Job drawing, mm, ordinate dimensions from the low corner. One solid piece. A direction names the side the tool comes from. Coordinates: 2 decimals unless noted, no trailing zeros. Write each loop counter-clockwise with the first axis right and the second up, starting at its lowest first coordinate (ties: lowest second). Pieces come first, ordered by that corner, then holes. Notation, with made-up numbers: (34.25, 49) -> (87.25, 49) arc R9 ccw to (87.25, 58) -> close; hole circle Ø7 at (-3.75, -38.5). An arc over 180 degrees is marked (long way). One line per question, with ' | ' between items. Start each with the question number.
Item 1: Saw through at B-B (z = 20). List the corners of the cut face in (x, y), and give its area (3 significant figures).
Item 2: Saw through at D-D (y = 4.5). List the corners of the cut face in (x, z), and give its area (3 significant figures).
Item 3: Two-plate mould, pull along Z, no slides. Class the marked faces 3, 4 and 5: pulls with the +Z half, pulls with the -Z half, needs draft (parallel to the pull), parting line crosses it, or undercut.
Item 4: Pin check, flat tips, straight feed: pin 1 (7 mm diameter, centred on x = 15, z = 20, fed in from +Y); pin 2 (2.5 mm diameter, centred on x = 89.5, y = 13.5, fed in from -Z); pin 3 (3.5 mm diameter, centred on x = 15, z = 20, fed in from -Y); pin 4 (4 mm diameter, centred on x = 129.5, z = 18, fed in from +Y). Stop position of each tip, or through.
Item 5: Probe probe 1 along Z at (x, y) = (74.5, 19); probe 2 along X at (y, z) = (9.25, 9); probe 3 along X at (y, z) = (17.5, 17.5). List the from-to ranges inside material, lowest first. Write a range as [from, to].
Item 6: Saw through at C-C (x = 135). List the corners of the cut face in (y, z), and give its area (3 significant figures).
Item 7: 3-axis set-ups, long thin cutter, end or side, ignore diameter. For the marked faces 1 and 2: which of +Z, -Z, +X, -X, +Y, -Y reach the whole face in a straight line?
Item 8: Saw through at A-A (y = 13.5). List the corners of the cut face in (x, z), and give its area (3 significant figures).
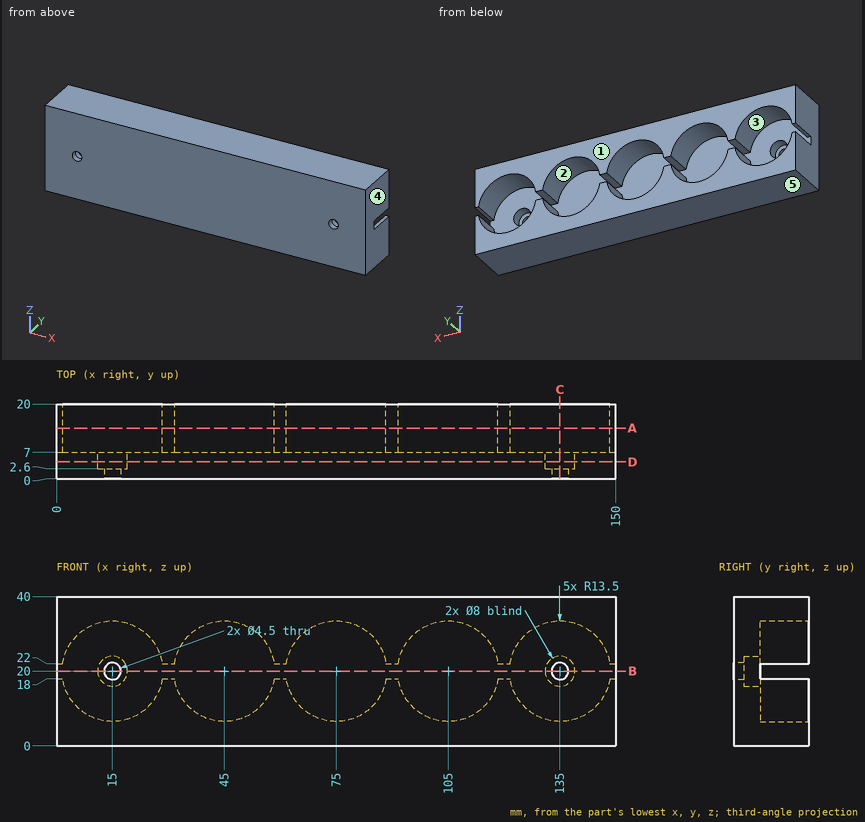
From the geometry:
1) outline: (0, 0) -> (12.75, 0) -> (12.75, 2.6) -> (11, 2.6) -> (11, 7) -> (0, 7) -> close; (17.25, 0) -> (132.75, 0) -> (132.75, 2.6) -> (131, 2.6) -> (131, 7) -> (19, 7) -> (19, 2.6) -> (17.25, 2.6) -> close; (137.25, 0) -> (150, 0) -> (150, 7) -> (139, 7) -> (139, 2.6) -> (137.25, 2.6) -> close | area: 956 mm2
2) outline: (0, 0) -> (150, 0) -> (150, 40) -> (0, 40) -> close; hole circle Ø8 at (15, 20); hole circle Ø8 at (135, 20) | area: 5,900 mm2
3) face 3: undercut | face 4: needs draft | face 5: pulls with the -Z half
4) pin 1: y = 2.6 | pin 2: z = 0 | pin 3: through | pin 4: y = 7
5) probe 1: [0, 6.51], [33.49, 40] | probe 2: [0, 7.17], [22.83, 37.17], [52.83, 67.17], [82.83, 97.17], [112.83, 127.17], [142.83, 150] | probe 3: [0, 1.73], [28.27, 31.73], [58.27, 61.73], [88.27, 91.73], [118.27, 121.73], [148.27, 150]
6) outline: (0, 0) -> (20, 0) -> (20, 6.5) -> (7, 6.5) -> (7, 16) -> (2.6, 16) -> (2.6, 17.75) -> (0, 17.75) -> close; (0, 22.25) -> (2.6, 22.25) -> (2.6, 24) -> (7, 24) -> (7, 33.5) -> (20, 33.5) -> (20, 40) -> (0, 40) -> close | area: 402 mm2
7) face 1: +Z, -Z, +X, -X, +Y | face 2: +Y
8) outline: (0, 0) -> (150, 0) -> (150, 18) -> (148.35, 18) arc R13.5 cw to (121.65, 18) -> (118.35, 18) arc R13.5 cw to (91.65, 18) -> (88.35, 18) arc R13.5 cw to (61.65, 18) -> (58.35, 18) arc R13.5 cw to (31.65, 18) -> (28.35, 18) arc R13.5 cw to (1.65, 18) -> (0, 18) -> close; (0, 22) -> (1.65, 22) arc R13.5 cw to (28.35, 22) -> (31.65, 22) arc R13.5 cw to (58.35, 22) -> (61.65, 22) arc R13.5 cw to (88.35, 22) -> (91.65, 22) arc R13.5 cw to (118.35, 22) -> (121.65, 22) arc R13.5 cw to (148.35, 22) -> (150, 22) -> (150, 40) -> (0, 40) -> close | area: 3,080 mm2
